Model file for the job. Use its own axes, mm. Face numbers are marked on the shaded views. A direction names the side the tool comes from. Coordinates: 2 decimals unless noted, no trailing zeros. Order: outer loops, then holes, each group sorted by start corner. A loop starts at its lowest first (then second) coordinate and runs counter-clockwise, first axis right, second up. Notation, with made-up numbers: (46, 26) -> (67, 26) arc R25 ccw to (67, 47) -> close; hole circle Ø1 at (43, 11.25). An arc over 180 degrees is marked (long way). Write item = value, one per line. Start each with the question number.
Q1. Cut at A-A, the plane y = 16. List the corners of the cut face in (x, z), plus the area to 3 significant figures.
Q2. Flat gauge pins, fed straight in: pin 1 (9.5 mm diameter, centred on y = 21, z = 29.5, fed in from -X); pin 2 (6 mm diameter, centred on x = -22.5, y = 13, fed in from +Z); pin 3 (4 mm diameter, centred on x = 0.5, y = 22.5, fed in from +Z). Where does each tip first touch, or does it go through?
Q3. Cut at D-D, the plane x = -12. List the corners of the cut face in (y, z), plus the area to 3 significant figures.
Q4. Cut at B-B, the plane z = 46. List the corners of the cut face in (x, y).
Q5. Cut at C-C, the plane z = 10. List the corners of the cut face in (x, y), plus the area to 3 significant figures.
Q6. Mould opens along Y. For the marked faces 6, 7, 8 and 9 say: +Y half, -Y half, draft (parallel to the pull), parting line (faces both ways), or undercut.
Q7. Wall check: line 1 (X direction, y = 3, z = 39); line 2 (Z direction, x = 2.5, y = 14); line 3 (X direction, y = 27, z = 5.5). Give the ranges that are in metal, low to high. Write a range as from..to.
Q8. 3-axis set-ups, long thin cutter, end or side, ignore diameter. For the marked faces 1, 2, 3, 4 and 5: which of +Z, -Z, +X, -X, +Y, -Y reach the whole face in a straight line?
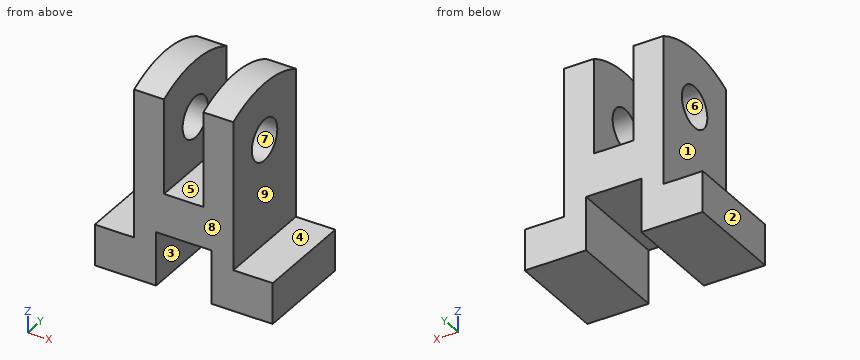
from build123d import *

# Parameters (mm, degrees)
F0_W     = 32
F0_H     = 13
F1_DEPTH = 28.25
F0_H_2   = 4
F0_R     = 6.5
F2_DEPTH = 15.75
F3_DEPTH = 6.25
F4_DEPTH = 8.75
F6_R     = 6.5
F7_DEPTH = 50


with BuildPart() as f1:
    # F0 (on Right) → F1 (new body, symmetric)
    with BuildSketch(Plane.YZ):
        with Locations((16, 6.5)):
            Rectangle(F0_W, F0_H)
    extrude(amount=F1_DEPTH, both=True)

    # F0 (on Right) → F2 (join, symmetric)
    with BuildSketch(Plane.YZ):
        with Locations((16, 23.5)):
            Rectangle(F0_W, F0_H)
        with Locations((16, 15)):
            Rectangle(F0_W, F0_H_2)
        with BuildLine():
            Line((0, 60.128765), (0, 30))
            Line((0, 30), (32, 30))
            Line((32, 30), (32, 60.128765))
            ThreePointArc((32, 60.128765), (16, 64), (0, 60.128765))
        make_face()
        with Locations((16, 46)):
            Circle(F0_R, mode=Mode.SUBTRACT)
    extrude(amount=F2_DEPTH, both=True)

    # F0 (on Right) → F3 (cut, symmetric)
    with BuildSketch(Plane.YZ):
        with BuildLine():
            Line((0, 60.128765), (0, 30))
            Line((0, 30), (32, 30))
            Line((32, 30), (32, 60.128765))
            ThreePointArc((32, 60.128765), (16, 64), (0, 60.128765))
        make_face()
        with Locations((16, 46)):
            Circle(F0_R, mode=Mode.SUBTRACT)
    extrude(amount=F3_DEPTH, both=True, mode=Mode.SUBTRACT)

    # F0 (on Right) → F4 (cut, symmetric)
    with BuildSketch(Plane.YZ):
        with Locations((16, 15)):
            Rectangle(F0_W, F0_H_2)
        with Locations((16, 6.5)):
            Rectangle(F0_W, F0_H)
    extrude(amount=F4_DEPTH, both=True, mode=Mode.SUBTRACT)


with BuildPart() as f7:
    # F6 (on offset) → F7 (new body)
    with BuildSketch(Plane(origin=(40.75, 16, 37.144454), x_dir=(0, 1, 0), z_dir=(1, 0, 0))):
        with Locations((16, 46)):
            Circle(F6_R)
    extrude(amount=F7_DEPTH)


solid = f1.part
Here are the results:
q1.outline = (-28.25, 0) -> (-8.75, 0) -> (-8.75, 17) -> (8.75, 17) -> (8.75, 0) -> (28.25, 0) -> (28.25, 13) -> (15.75, 13) -> (15.75, 39.5) -> (6.25, 39.5) -> (6.25, 30) -> (-6.25, 30) -> (-6.25, 39.5) -> (-15.75, 39.5) -> (-15.75, 13) -> (-28.25, 13) -> close; (-15.75, 52.5) -> (-6.25, 52.5) -> (-6.25, 64) -> (-15.75, 64) -> close; (6.25, 52.5) -> (15.75, 52.5) -> (15.75, 64) -> (6.25, 64) -> close
q1.area = 1,370 mm²
q2.pin_1 = -15.75
q2.pin_2 = 13
q2.pin_3 = 30
q3.outline = (0, 0) -> (32, 0) -> (32, 60.13) arc R35 ccw to (0, 60.13) -> close; hole circle Ø13 at (16, 46)
q3.area = 1,870 mm²
q4.outline = (-15.75, 0) -> (-6.25, 0) -> (-6.25, 9.5) -> (-15.75, 9.5) -> close; (-15.75, 22.5) -> (-6.25, 22.5) -> (-6.25, 32) -> (-15.75, 32) -> close; (6.25, 0) -> (15.75, 0) -> (15.75, 9.5) -> (6.25, 9.5) -> close; (6.25, 22.5) -> (15.75, 22.5) -> (15.75, 32) -> (6.25, 32) -> close
q5.outline = (-28.25, 0) -> (-8.75, 0) -> (-8.75, 32) -> (-28.25, 32) -> close; (8.75, 0) -> (28.25, 0) -> (28.25, 32) -> (8.75, 32) -> close
q5.area = 1,250 mm²
q6.face_6 = undercut
q6.face_7 = undercut
q6.face_8 = -Y half
q6.face_9 = draft
q7.line_1 = -15.75..-6.25, 6.25..15.75
q7.line_2 = 17..30
q7.line_3 = -28.25..-8.75, 8.75..28.25
q8.face_1 = +Z, -X, +Y, -Y
q8.face_2 = +Z, -Z, -X, +Y, -Y
q8.face_3 = -Z, +Y, -Y
q8.face_4 = +Z, +X, +Y, -Y
q8.face_5 = +Z, +Y, -Y
